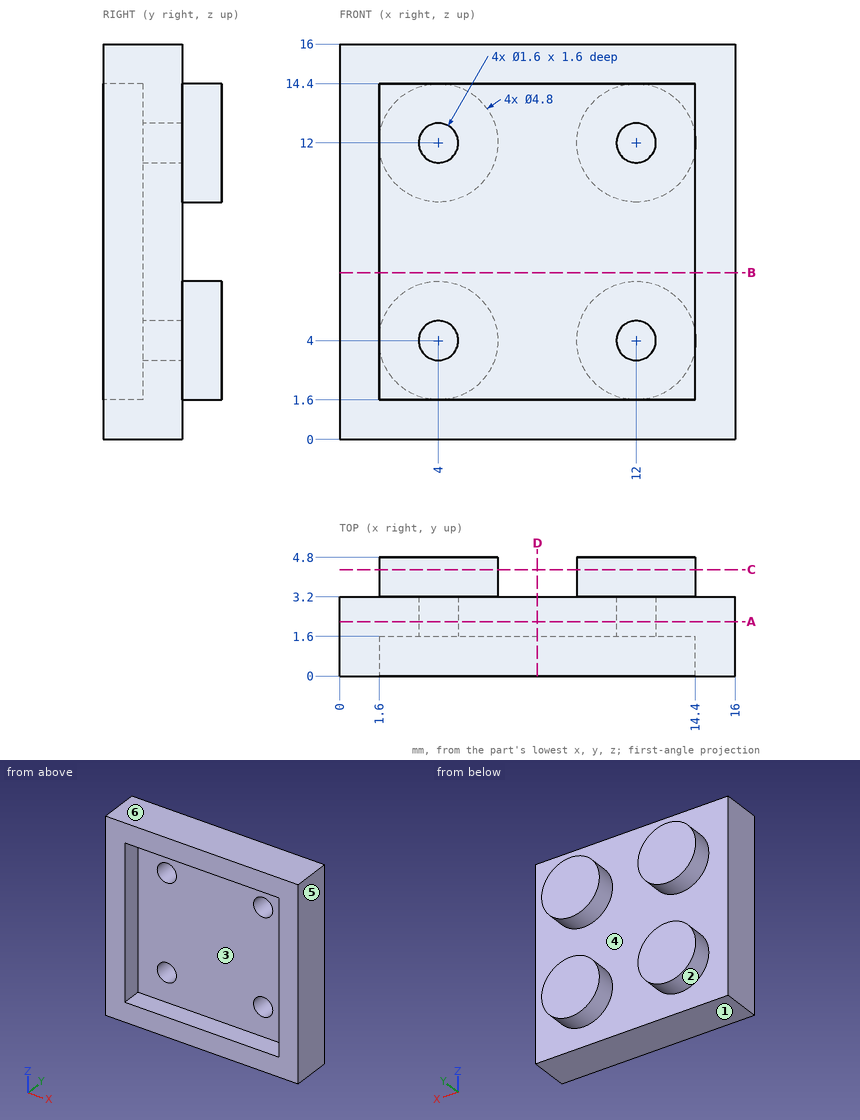
Input: dimensioned drawing with shaded views. Units: mm. Origin: part minimum x, y, z. A direction names the side the tool comes from. Coordinates: 2 decimals unless noted, no trailing zeros. Order: outer loops, then holes, each group sorted by start corner. A loop starts at its lowest first (then second) coordinate and runs counter-clockwise, first axis right, second up. Notation, with made-up numbers: (-25, 7.5) -> (9, 7.5) arc R34 cw to (9, 43.5) -> close; hole circle Ø7 at (34, 48.5). An arc over 180 degrees is marked (long way). Answer in a Markdown table with one row per item.
Item 1: Section D-D on x = 8. Output: boundary loops of the cut face in (y, z).
Return value:
| item | result |
|---|---|
| outline | (0, 0) -> (3.2, 0) -> (3.2, 16) -> (0, 16) -> (0, 14.4) -> (1.6, 14.4) -> (1.6, 1.6) -> (0, 1.6) -> close |
Item 2: Section C-C on y = 4.3. Output: boundary loops of the cut face in (x, z).
Return value:
| item | result |
|---|---|
| outline | circle Ø4.8 at (4, 4); circle Ø4.8 at (4, 12); circle Ø4.8 at (12, 4); circle Ø4.8 at (12, 12) |
Item 3: Access query for the marked faces 1 and 2. Directions: +Z, -Z, +X, -X, +Y, -Y. A direction counts if a zero-diameter tool reaches every point of the face in a straight line with its end or side. Return the directions, or none.
Return value:
| item | result |
|---|---|
| face 1 | -Z, +X, -X, +Y, -Y |
| face 2 | +Y |
Item 4: Ray query, L1, parallel to X at y = 2.1, z = 12; L2, parallel to Z at x = 8, y = 0.5. Return the intervals inside material, ascending.
Return value:
| item | result |
|---|---|
| L1 | x = 0 to 3.2, 4.8 to 11.2, 12.8 to 16 |
| L2 | z = 0 to 1.6, 14.4 to 16 |
Item 5: Draft query along Z for the marked faces 3, 4, 5 and 6. Return one class per face: released by +Z, released by -Z, zero draft, split by the parting line, or undercut.
Return value:
| item | result |
|---|---|
| face 3 | undercut |
| face 4 | undercut |
| face 5 | zero draft |
| face 6 | released by +Z |
Item 6: Section B-B on z = 6.75. Output: boundary loops of the cut face in (x, y), plus the area to 3 significant figures.
Return value:
| item | result |
|---|---|
| outline | (0, 0) -> (1.6, 0) -> (1.6, 1.6) -> (14.4, 1.6) -> (14.4, 0) -> (16, 0) -> (16, 3.2) -> (0, 3.2) -> close |
| area | 30.7 mm² |
Item 7: Contact query for flat-ended pins moving along their axis: P1, Ø0.8, axis at x = 11.5, z = 12.5, coming from the -Y side; P2, Ø0.5, axis at x = 4, z = 4, coming from the -Y side. Output: stop coordinate, or through.
Return value:
| item | result |
|---|---|
| P1 | stops at y = 1.6 |
| P2 | stops at y = 3.2 |
Item 8: Section A-A on y = 2.2. Output: boundary loops of the cut face in (x, z), plus the area to 3 significant figures.
Return value:
| item | result |
|---|---|
| outline | (0, 0) -> (16, 0) -> (16, 16) -> (0, 16) -> close; hole circle Ø1.6 at (4, 4); hole circle Ø1.6 at (4, 12); hole circle Ø1.6 at (12, 4); hole circle Ø1.6 at (12, 12) |
| area | 248 mm² |
